The listing builds one solid part. Answer for the finished solid, in the listing's coordinates (mm). Coordinates: 2 decimals unless noted, no trailing zeros. Order: outer loops, then holes, each group sorted by start corner. A loop starts at its lowest first (then second) coordinate and runs counter-clockwise, first axis right, second up. Notation, with made-up numbers: M 55.25,39 L 106.25,39 A25 cw 106.25,59 Z; hole C -37.75,48.5 d9. An arc over 180 degrees is marked long. One line per item, written item: value. Start each with the question number.
Q1. The part is cut by section C-C on x = -4.5. Give the vertices of the cut face in (y, z), then the cut area to 3 significant figures.
Q2. Straight lines are drawn through the part: line 1 along X through (y, z) = (47, -5); line 2 along Z through (x, y) = (3.5, 45); line 3 along X through (y, z) = (6, -2). For each, find the intervals that lie inside material, in ascending order. Write a range as [from, to].
Q3. The part is cut by section A-A on y = 27. Give the vertices of the cut face in (x, z), then the cut area to 3 significant figures.
Q4. The part is cut by section B-B on z = -3.5. Give the vertices of the cut face in (x, y).
Q5. Each of these flat-tipped pins is pushed along its axis until it touches: pin 1 Ø3 at (y, z) = (36, 3) entering from +X; pin 2 Ø5 at (x, y) = (-4.5, 31) entering from +Z. Where does it stop, or does it pass through?
Q6. The part is cut by section D-D on x = 2.5. Give the vertices of the cut face in (y, z).
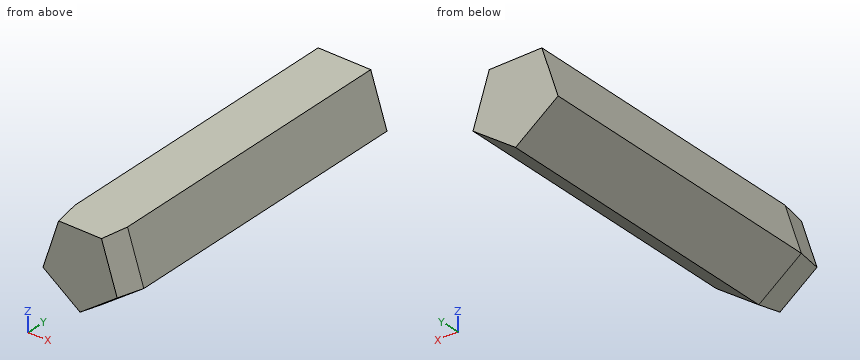
```python
from build123d import *
from OCP.BRepFilletAPI import BRepFilletAPI_MakeChamfer

# Parameters (mm, degrees)
BOSS_EXTRUDE1_DEPTH = 50
CHAMFER1_SIZE       = 4
CHAMFER1_SIZE2      = 0.705307923


with BuildPart() as part:
    # Sketch1 → Boss-Extrude1 (new body)
    with BuildSketch(Plane(origin=(0, 0, 0), x_dir=(1, 0, 0), z_dir=(0, 1, 0))):
        Polygon((0, 6.771180434), (-6.439775275, 2.092409826), (-3.98, -5.478000043), (3.98, -5.478000043), (6.439775275, 2.092409826), align=None)
    extrude(amount=BOSS_EXTRUDE1_DEPTH)

    # Chamfer1: one chamfer whose edges measure the first distance from different faces: ONE call of the kernel's chamfer builder (chamfer() names one face for all edges)
    chamfer1_edges_1 = [part.edges().sort_by_distance(p)[0] for p in [
        (5.209887638, 0, 1.692795109),
    ]]
    chamfer1_side_1 = [part.faces().sort_by_distance(p)[0] for p in [
        (5.209887638, 25, 1.692795109),
    ]]
    chamfer1_edges_2 = [part.edges().sort_by_distance(p)[0] for p in [
        (-5.209887638, 0, 1.692795109),
    ]]
    chamfer1_side_2 = [part.faces().sort_by_distance(p)[0] for p in [
        (-5.209887638, 25, 1.692795109),
    ]]
    chamfer1_edges_3 = [part.edges().sort_by_distance(p)[0] for p in [
        (-3.219887638, 0, -4.43179513),
    ]]
    chamfer1_side_3 = [part.faces().sort_by_distance(p)[0] for p in [
        (-3.219887638, 25, -4.43179513),
    ]]
    chamfer1_edges_4 = [part.edges().sort_by_distance(p)[0] for p in [
        (3.219887638, 0, -4.43179513),
    ]]
    chamfer1_side_4 = [part.faces().sort_by_distance(p)[0] for p in [
        (3.219887638, 25, -4.43179513),
    ]]
    chamfer1 = BRepFilletAPI_MakeChamfer(part.part.solid().wrapped)
    for e in chamfer1_edges_1:
        chamfer1.Add(CHAMFER1_SIZE, CHAMFER1_SIZE2, e.wrapped, chamfer1_side_1[0].wrapped)  # the first distance lies on this face
    for e in chamfer1_edges_2:
        chamfer1.Add(CHAMFER1_SIZE, CHAMFER1_SIZE2, e.wrapped, chamfer1_side_2[0].wrapped)  # the first distance lies on this face
    for e in chamfer1_edges_3:
        chamfer1.Add(CHAMFER1_SIZE, CHAMFER1_SIZE2, e.wrapped, chamfer1_side_3[0].wrapped)  # the first distance lies on this face
    for e in chamfer1_edges_4:
        chamfer1.Add(CHAMFER1_SIZE, CHAMFER1_SIZE2, e.wrapped, chamfer1_side_4[0].wrapped)  # the first distance lies on this face
    add(Compound.cast(chamfer1.Shape()), mode=Mode.REPLACE)


solid = part.part
```
Output:
1. outline: M 0,-2.63 L 4,-3.5 L 50,-3.5 L 50,3.88 L 4,3.88 L 0,1.6 Z
1. area: 363 mm^2
2. line 1: x = [-2.44, 2.44]
2. line 2: z = [-4.23, 5.48]
2. line 3: x = [-6.41, 6.41]
3. outline: M -6.44,-2.09 L 0,-6.77 L 6.44,-2.09 L 3.98,5.48 L -3.98,5.48 Z
3. area: 109 mm^2
4. outline: M -4.5,4 L -3.3,0 L 3.3,0 L 4.5,4 L 4.5,50 L -4.5,50 Z
5. pin 1: stops at x = 5.27
5. pin 2: stops at z = 5.48
6. outline: M 0,-4.08 L 4,-4.95 L 50,-4.95 L 50,5.48 L 0,5.48 Z
